from build123d import *

# Parameters (mm, degrees)
SKETCH1_W           = 600
SKETCH1_H           = 600
BOSS_EXTRUDE1_DEPTH = 1000
SKETCH1_3_W         = 600
SKETCH1_3_H         = 600
BOSS_EXTRUDE2_DEPTH = 1000


with BuildPart() as part:
    # Sketch1 → Boss-Extrude1 (new body)
    with BuildSketch(Plane(origin=(0, 0, 0), x_dir=(1, 0, 0), z_dir=(0, 1, 0))):
        Polygon((200, 800), (-200, 800), (-200, 200), (-800, 200), (-800, -200), (200, -200), align=None)
        with Locations((-500, 500)):
            Rectangle(SKETCH1_W, SKETCH1_H)
    extrude(amount=-BOSS_EXTRUDE1_DEPTH)

    # Sketch1_3 → Boss-Extrude2 (add)
    with BuildSketch(Plane(origin=(0, 0, 0), x_dir=(1, 0, 0), z_dir=(0, 1, 0))):
        with Locations((-500, 500)):
            Rectangle(SKETCH1_3_W, SKETCH1_3_H)
    extrude(amount=BOSS_EXTRUDE2_DEPTH)


solid = part.part
Geometry check sheet. Reference: the model listing, model coordinates, mm. A direction names the side the tool comes from. Give positions to 0.01 mm unless a question says otherwise; leave off trailing zeros. Loops run counter-clockwise (first coordinate to the right, second up) from the corner with the lowest first, then second, coordinate; pieces in that order, holes last. Notation, with made-up numbers: (46.5, -8.75) -> (56.5, -8.75) arc R31 ccw to (56.5, 15.25) -> close; hole circle Ø9 at (8.25, 53). An arc over 180 degrees is marked (long way). Answer in a Markdown table with one row per item. Add a question column.
1) Set-up check for faces 1 (the face through (-200, 493, -496)), 2 (the face through (-504, 493, -200)), 3 (the face through (-307, -1000, -307)): record each of +Z, -Z, +X, -X, +Y, -Y from which the full face is reachable in a straight line by a thin tool's end or side.
2) Gauge pin test, flat end, axial feed: P1, Ø2, axis at x = -40.5, z = -449, coming from the +Y side. Record the tip position at first contact, or that the pin passes through.
3) Cross-section at A-A on x = 131. Record the boundary of the cut face in (y, z), and give its area (3 significant figures).
4) Cross-section at B-B on z = -731.5. Record the boundary of the cut face in (x, y), and give its area (3 significant figures).
5) Cross-section at D-D on x = -264.5. Record the boundary of the cut face in (y, z).
6) Cross-section at C-C on y = 412.5. Record the boundary of the cut face in (x, z).
7) Material ranges on probe 1 along X at (y, z) = (450.5, -203); probe 2 along Y at (x, z) = (9.5, -555), recorded low to high. Write a range as from..to.
Outcome:
| question | item | result |
|---|---|---|
| 1 | face 1 | +Z, -Z, +X, +Y |
| 1 | face 2 | +Z, +X, -X, +Y |
| 1 | face 3 | +Z, -Z, +X, -X, -Y |
| 2 | P1 | stops at y = 0 |
| 3 | outline | (-1000, -800) -> (0, -800) -> (0, 200) -> (-1000, 200) -> close |
| 3 | area | 1,000,000 mm^2 |
| 4 | outline | (-800, -1000) -> (200, -1000) -> (200, 0) -> (-200, 0) -> (-200, 1000) -> (-800, 1000) -> close |
| 4 | area | 1,600,000 mm^2 |
| 5 | outline | (-1000, -800) -> (1000, -800) -> (1000, -200) -> (0, -200) -> (0, 200) -> (-1000, 200) -> close |
| 6 | outline | (-800, -800) -> (-200, -800) -> (-200, -200) -> (-800, -200) -> close |
| 7 | probe 1 | x = -800..-200 |
| 7 | probe 2 | y = -1000..0 |
